from build123d import *

# Parameters (mm, degrees)
ESQUISSE1_W        = 5
ESQUISSE1_H        = 5
BOSS_EXTRU_1_DEPTH = 25


with BuildPart() as part:
    # Esquisse1 → Boss.-Extru.1 (new, symmetric)
    with BuildSketch(Plane.XY):
        with BuildLine():
            Line((25.022912308, -13.003609484), (4.817627458, -1.338082837))
            ThreePointArc((4.817627458, -1.338082837), (5, 0), (4.817627458, 1.338082837))
            Line((4.817627458, 1.338082837), (25.022912308, 13.003609484))
            ThreePointArc((25.022912308, 13.003609484), (24.421916387, 14.1), (23.772912308, 15.168672994))
            Line((23.772912308, 15.168672994), (3.567627458, 3.503146346))
            ThreePointArc((3.567627458, 3.503146346), (2.5, 4.330127019), (1.25, 4.841229183))
            Line((1.25, 4.841229183), (1.25, 28.172282478))
            ThreePointArc((1.25, 28.172282478), (0, 28.2), (-1.25, 28.172282478))
            Line((-1.25, 28.172282478), (-1.25, 4.841229183))
            ThreePointArc((-1.25, 4.841229183), (-2.5, 4.330127019), (-3.567627458, 3.503146346))
            Line((-3.567627458, 3.503146346), (-23.772912308, 15.168672994))
            ThreePointArc((-23.772912308, 15.168672994), (-24.421916387, 14.1), (-25.022912308, 13.003609484))
            Line((-25.022912308, 13.003609484), (-4.817627458, 1.338082837))
            ThreePointArc((-4.817627458, 1.338082837), (-5, 0), (-4.817627458, -1.338082837))
            Line((-4.817627458, -1.338082837), (-25.022912308, -13.003609484))
            ThreePointArc((-25.022912308, -13.003609484), (-24.421916387, -14.1), (-23.772912308, -15.168672994))
            Line((-23.772912308, -15.168672994), (-3.567627458, -3.503146346))
            ThreePointArc((-3.567627458, -3.503146346), (-2.5, -4.330127019), (-1.25, -4.841229183))
            Line((-1.25, -4.841229183), (-1.25, -28.172282478))
            ThreePointArc((-1.25, -28.172282478), (0, -28.2), (1.25, -28.172282478))
            Line((1.25, -28.172282478), (1.25, -4.841229183))
            ThreePointArc((1.25, -4.841229183), (2.5, -4.330127019), (3.567627458, -3.503146346))
            Line((3.567627458, -3.503146346), (23.772912308, -15.168672994))
            ThreePointArc((23.772912308, -15.168672994), (24.421916387, -14.1), (25.022912308, -13.003609484))
        make_face()
        Rectangle(ESQUISSE1_W, ESQUISSE1_H, mode=Mode.SUBTRACT)
    extrude(amount=BOSS_EXTRU_1_DEPTH, both=True)


solid = part.part
Input: part model. Units: mm. Frame: model coordinates. A direction names the side the tool comes from. Give positions to 0.01 mm unless a question says otherwise; leave off trailing zeros. Order: outer loops, then holes, each group sorted by start corner. A loop starts at its lowest first (then second) coordinate and runs counter-clockwise, first axis right, second up. Notation, with made-up numbers: (58, 67) - (83, 67) arc R8 cw to (83, 78) - close; hole circle Ø10 at (68.5, -6). An arc over 180 degrees is marked (long way). Write each question's results on one line, items separated by ' | '.
Item 1: Draft query along Y for faces 6 (the flat face through (0, 2.5, 0)), 7 (the flat face through (4, 0, 25)), 8 (the cylindrical face through (-24.431, -14.085, 0.35)). Return one class per face: released by +Y, released by -Y, zero draft, split by the parting line, or undercut.
A:
face 6: undercut | face 7: zero draft | face 8: released by -Y
Item 2: Section C-C (x = -10.5). Return loops of the section in (y, z), and give its area (3 significant figures).
A:
outline: (-7.51, -25) - (-4.62, -25) - (-4.62, 25) - (-7.51, 25) - close; (4.62, -25) - (7.51, -25) - (7.51, 25) - (4.62, 25) - close | area: 289 mm^2
Item 3: Section D-D (y = -24). Return loops of the section in (x, z).
A:
outline: (-1.25, -25) - (1.25, -25) - (1.25, 25) - (-1.25, 25) - close
Item 4: Section A-A (z = 3). Return loops of the section in (x, y).
A:
outline: (-25.02, -13) arc R28.2 ccw to (-23.77, -15.17) - (-3.57, -3.5) arc R5 ccw to (-1.25, -4.84) - (-1.25, -28.17) arc R28.2 ccw to (1.25, -28.17) - (1.25, -4.84) arc R5 ccw to (3.57, -3.5) - (23.77, -15.17) arc R28.2 ccw to (25.02, -13) - (4.82, -1.34) arc R5 ccw to (4.82, 1.34) - (25.02, 13) arc R28.2 ccw to (23.77, 15.17) - (3.57, 3.5) arc R5 ccw to (1.25, 4.84) - (1.25, 28.17) arc R28.2 ccw to (-1.25, 28.17) - (-1.25, 4.84) arc R5 ccw to (-3.57, 3.5) - (-23.77, 15.17) arc R28.2 ccw to (-25.02, 13) - (-4.82, 1.34) arc R5 ccw to (-4.82, -1.34) - close; hole (-2.5, -2.5) - (2.5, -2.5) - (2.5, 2.5) - (-2.5, 2.5) - close
Item 5: Section B-B (y = 14). Return loops of the section in (x, z), and give its area (3 significant figures).
A:
outline: (-24.48, -25) - (-21.75, -25) - (-21.75, 25) - (-24.48, 25) - close; (-1.25, -25) - (1.25, -25) - (1.25, 25) - (-1.25, 25) - close; (21.75, -25) - (24.48, -25) - (24.48, 25) - (21.75, 25) - close | area: 398 mm^2
Item 6: Access query for faces 1 (the flat face through (15.06, -7.25, 0.35)), 2 (the cylindrical face through (2.48, -4.34, 0.35)), 3 (the flat face through (0, -2.5, 0)), 4 (the cylindrical face through (3, 4, 0)), 5 (the cylindrical face through (24.41, -14.12, 0.35)). Directions: +Z, -Z, +X, -X, +Y, -Y. A direction counts if a zero-diameter tool reaches every point of the face in a straight line with its end or side. Return the directions, or none.
A:
face 1: +Z, -Z, +X | face 2: +Z, -Z, -Y | face 3: +Z, -Z | face 4: +Z, -Z, +Y | face 5: +Z, -Z, +X, -Y
Item 7: Contact query for flat-ended pins moving along their axis: pin 1 Ø10 at (x, z) = (-9.5, 16) entering from +Y; pin 2 Ø7 at (y, z) = (-22, 1.5) entering from -X; pin 3 Ø7 at (y, z) = (16, -2) entering from +X; pin 4 Ø10 at (x, y) = (-9.5, -18.5) entering from -Z. Output: stop coordinate, or through.
A:
pin 1: stops at y = 9.81 | pin 2: stops at x = -1.25 | pin 3: stops at x = 25.02 | pin 4: passes through
Item 8: Material intervals for line 1 along X through (y, z) = (-13, 7); line 2 along X through (y, z) = (-13.5, -12); line 3 along X through (y, z) = (20, 14), sorted ascending.
A:
line 1: x = -25.02 to -20.02, -1.25 to 1.25, 20.02 to 25.02 | line 2: x = -24.76 to -20.88, -1.25 to 1.25, 20.88 to 24.76 | line 3: x = -1.25 to 1.25
